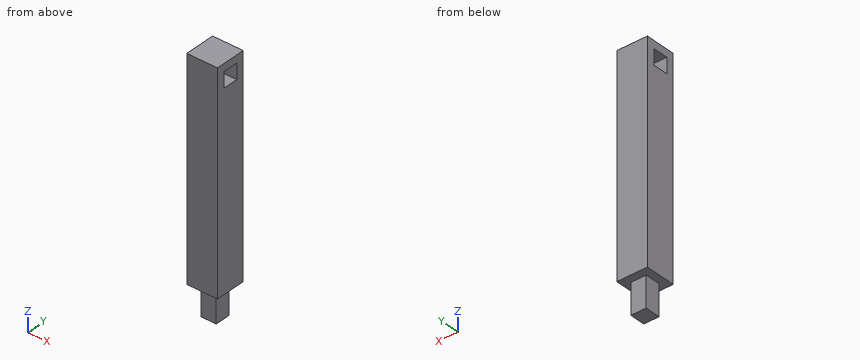
Autodesk Inventor part; units mm, degrees
ref_plane "YZ Plane" through (0, 0, 0) normal (1, 0, 0) x (0, 1, 0)
ref_plane "XZ Plane" through (0, 0, 0) normal (0, 1, 0) x (-1, 0, 0)
ref_plane "XY Plane" through (0, 0, 0) normal (0, 0, 1) x (1, 0, 0)
sketch "Sketch1" plane through (0, 0, 0) normal (1, 0, 0) x (0, 1, 0)
  line L0 (0, 0) -> (25.4, 0)
  line L1 (25.4, 0) -> (25.4, -203.2)
  line L2 (25.4, -203.2) -> (0, -203.2)
  line L3 (0, -203.2) -> (0, 0)
  line L4 (19.05, -6.35) -> (6.35, -6.35)
  line L5 (6.35, -6.35) -> (6.35, -19.05)
  line L6 (6.35, -19.05) -> (19.05, -19.05)
  line L7 (19.05, -19.05) -> (19.05, -6.35)
  dimension "d0" = 25.4
  dimension "d1" = 203.2
  dimension "d2" = 12.7
  dimension "d3" = 12.7
  dimension "d4" = 6.35
  dimension "d5" = 6.35
extrude "Extrusion1" add sketch "Sketch1" along normal blind 25.4
sketch "Sketch2" plane through (0, 0, -203.2) normal (0, 0, -1) x (-1, 0, 0)
  point P0 (0, 0)
sketch "Sketch3" plane through (0, 0, -203.2) normal (0, 0, -1) x (-1, 0, 0)
  line L0 (-19.05, 19.05) -> (-6.35, 19.05)
  line L1 (-6.35, 19.05) -> (-6.35, 6.35)
  line L2 (-6.35, 6.35) -> (-19.05, 6.35)
  line L3 (-19.05, 6.35) -> (-19.05, 19.05)
  line L4 (0, 25.4) -> (0, 0)
  line L5 (0, 25.4) -> (-25.4, 25.4)
  line L6 (-25.4, 0) -> (-25.4, 25.4)
  line L7 (0, 0) -> (-25.4, 0)
  dimension "d8" = 12.7
  dimension "d9" = 12.7
  dimension "d10" = 6.35
  dimension "d11" = 6.35
extrude "Extrusion2" cut sketch "Sketch3" against normal blind 25.4
equation "\"d9\" = d8"
properties part number "FrameAnalysisPart"
Work out the finished part from the listing and answer in its coordinate system (mm). Round coordinates to 2 decimals unless told otherwise and drop trailing zeros. Order: outer loops, then holes, each group sorted by start corner. A loop starts at its lowest first (then second) coordinate and runs counter-clockwise, first axis right, second up. Notation, with made-up numbers: M 86,57 L 112,57 A4 ccw 112,63 Z; hole C -38,-31 d7. An arc over 180 degrees is marked long. Put each result on its own line as item: value. Start each with the question number.
Q1. Section C-C, the plane y = 23.5 is taken. Write down the section's boundary in (x, z).
Q2. Section B-B, the plane x = 3.5 is taken. Write down the section's boundary in (y, z), and give its area (3 significant figures).
Q3. Straight lines are drawn through the part: L1, parallel to Z at x = 19.5, y = 6.5; L2, parallel to Z at x = 13.5, y = 15.5; L3, parallel to Y at x = 17, z = -16. For each, find the intervals that lie inside material, in ascending order. Write a range as [from, to].
Q4. Section A-A, the plane y = 10.25 is taken. Write down the section's boundary in (x, z).
Q5. Flat-ended cylindrical pins translate along their axes: pin 1 (4 mm diameter, centred on y = 8.5, z = -162, fed in from -X); pin 2 (10 mm diameter, centred on y = 15.5, z = -185.5, fed in from -X); pin 3 (6.5 mm diameter, centred on x = 11, z = -188, fed in from -Y); pin 4 (10 mm diameter, centred on x = 12, z = -191.5, fed in from +Y). Find the tip coordinate at first contact, or state that the pin passes through.
Findings below:
1. outline: M 0,-177.8 L 25.4,-177.8 L 25.4,0 L 0,0 Z
2. outline: M 0,-177.8 L 25.4,-177.8 L 25.4,0 L 0,0 Z; hole M 6.35,-19.05 L 19.05,-19.05 L 19.05,-6.35 L 6.35,-6.35 Z
2. area: 4,350 mm^2
3. L1: z = [-177.8, -19.05], [-6.35, 0]
3. L2: z = [-203.2, -19.05], [-6.35, 0]
3. L3: y = [0, 6.35], [19.05, 25.4]
4. outline: M 0,-177.8 L 6.35,-177.8 L 6.35,-203.2 L 19.05,-203.2 L 19.05,-177.8 L 25.4,-177.8 L 25.4,-19.05 L 0,-19.05 Z; M 0,-6.35 L 25.4,-6.35 L 25.4,0 L 0,0 Z
5. pin 1: stops at x = 0
5. pin 2: stops at x = 6.35
5. pin 3: stops at y = 6.35
5. pin 4: stops at y = 19.05
